Design review of the part built by this model. Coordinates are the model's own, in mm. Coordinates: 2 decimals unless noted, no trailing zeros. Loops run counter-clockwise (first coordinate to the right, second up) from the corner with the lowest first, then second, coordinate; pieces in that order, holes last. Notation, with made-up numbers: M -37.5,-38.75 L 4.5,-38.75 A8 ccw 4.5,-28.75 Z; hole C 38,-25 d9. An arc over 180 degrees is marked long. Answer as a JSON object with one key per item and string values. Group by question number.
1. Draft analysis for pull direction Z (two halves, no side actions). For faces 1 (the cylindrical face through (-2.75, -12.52, -12.4)), 2 (the flat face through (-62.73, -13, 1)), 3 (the flat face through (-13, -13, 20.359)), state which applies: +Z half, -Z half, draft (parallel to the pull), parting line (faces both ways), or undercut.
2. Consider section D-D (z = 6.5). State the section outline as (x, y) points, then the cut area to 3 significant figures.
3. Consider section A-A (z = 0). State the section outline as (x, y) points, then the cut area to 3 significant figures.
4. To check wall thickness, follow probe 1 along X at (y, z) = (-9, 9); probe 2 along X at (y, z) = (-6, 6); probe 3 along Z at (x, y) = (0, -20). State the ranges of each line that lie inside material, in increasing order.
5. Consider section C-C (y = -7.25). State the section outline as (x, z) points, then the cut area to 3 significant figures.
6. Insertion check: pin 1 (8 mm diameter, centred on x = 12, z = 2.5, fed in from +Y). The pin has a flat end and moves straight along its axis. Give the tip position at first contact, or say it passes through.
7. Consider section B-B (x = 0). State the section outline as (y, z) points, then the cut area to 3 significant figures.
from build123d import *

# Parameters (mm, degrees)
F0_W     = 101.6
F0_H     = 38.1
F0_R     = 12.7
F1_DEPTH = 25.4


with BuildPart() as f1:
    # F0 (on Front) → F1 (new body)
    with BuildSketch(Plane.XZ):
        with Locations((-11.930157, 1.308589)):
            Rectangle(F0_W, F0_H)
        with Locations((-46.90408, 0)):
            Circle(F0_R, mode=Mode.SUBTRACT)
        Circle(F0_R, mode=Mode.SUBTRACT)
    extrude(amount=F1_DEPTH)


solid = f1.part
Findings below:
{
 "1": {"face 1": "undercut", "face 2": "draft", "face 3": "+Z half"},
 "2": {"outline": "M -62.73,-25.4 L -57.81,-25.4 L -57.81,0 L -62.73,0 Z; M -35.99,-25.4 L -10.91,-25.4 L -10.91,0 L -35.99,0 Z; M 10.91,-25.4 L 38.87,-25.4 L 38.87,0 L 10.91,0 Z", "area": "1,470 mm^2"},
 "3": {"outline": "M -62.73,-25.4 L -59.6,-25.4 L -59.6,0 L -62.73,0 Z; M -34.2,-25.4 L -12.7,-25.4 L -12.7,0 L -34.2,0 Z; M 12.7,-25.4 L 38.87,-25.4 L 38.87,0 L 12.7,0 Z", "area": "1,290 mm^2"},
 "4": {"probe 1": "x = -62.73 to -55.86, -37.94 to -8.96, 8.96 to 38.87", "probe 2": "x = -62.73 to -58.1, -35.71 to -11.19, 11.19 to 38.87", "probe 3": "z = -17.74 to -12.7, 12.7 to 20.36"},
 "5": {"outline": "M -62.73,-17.74 L 38.87,-17.74 L 38.87,20.36 L -62.73,20.36 Z; hole C -46.9,0 d25.4; hole C 0,0 d25.4", "area": "2,860 mm^2"},
 "6": {"pin 1": "stops at y = 0"},
 "7": {"outline": "M -25.4,-17.74 L 0,-17.74 L 0,-12.7 L -25.4,-12.7 Z; M -25.4,12.7 L 0,12.7 L 0,20.36 L -25.4,20.36 Z", "area": "323 mm^2"}
}
